Could you check a few things on this model? Use its own coordinates, in mm. Face numbers are marked on the shaded views. A direction names the side the tool comes from. Give positions to 0.01 mm unless a question says otherwise; leave off trailing zeros. Order: outer loops, then holes, each group sorted by start corner. A loop starts at its lowest first (then second) coordinate and runs counter-clockwise, first axis right, second up. Notation, with made-up numbers: M 1,-30 L 28,-30 A33 ccw 28,7 Z; hole C 89,15 d10. An arc over 180 degrees is marked long. Use a Markdown table: item, result. Add a question column.
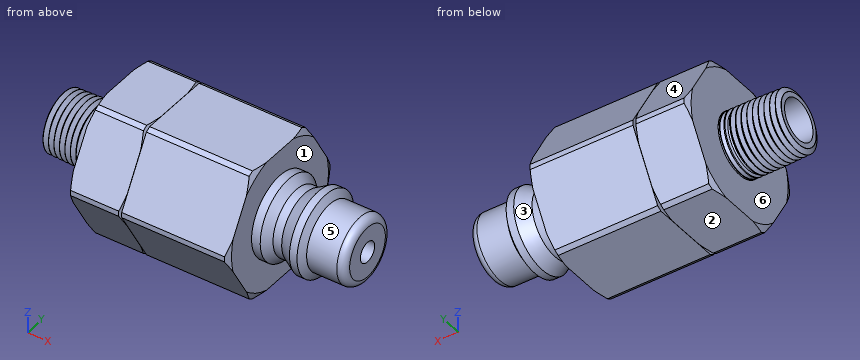
```python
from build123d import *

# Parameters (mm, degrees)
SKETCH6_W      = 11.300333551
SKETCH6_H      = 15.496408613
EXTRUDE1_DEPTH = 26.86304
FILLET1_R      = 1.27


with BuildPart() as part:
    # Sketch1 → Revolve1 (revolve)
    with BuildSketch(Plane.XY):
        Polygon((0, 0), (0, 4.202548436), (0.016953331, 4.234153018), (0.42773912, 4.999944315), (0.463586157, 5.001064591), (0.921387979, 4.262418014), (0.957235016, 4.26353829), (1.368020805, 5.029329586), (1.403867842, 5.030449862), (1.861669664, 4.291803285), (1.897516701, 4.292923561), (2.30830249, 5.058714857), (2.344149527, 5.059835133), (2.801951349, 4.321188556), (2.837798386, 4.322308832), (3.248584175, 5.088100128), (3.284431212, 5.089220404), (3.742233034, 4.350573827), (3.778080071, 4.351694103), (4.18886586, 5.1174854), (4.224712897, 5.118605675), (4.682514719, 4.379959098), (4.718361756, 4.381079374), (5.129147545, 5.146870671), (5.164994582, 5.147990947), (5.622796404, 4.409344369), (5.658643441, 4.410464645), (6.06942923, 5.176255942), (6.105276267, 5.177376218), (6.563078089, 4.43872964), (6.598925126, 4.439849916), (7.009710915, 5.205641213), (7.045557952, 5.206761489), (7.503359774, 4.468114911), (7.539206811, 4.469235187), (7.9499926, 5.235026484), (7.985839637, 5.23614676), (8.443641459, 4.497500182), (8.479488496, 4.498620458), (8.890274285, 5.264411755), (8.926121322, 5.265532031), (9.383923144, 4.526885454), (9.419770181, 4.528005729), (9.83055597, 5.293797026), (9.866403007, 5.294917302), (10.324204829, 4.556270725), (10.360051866, 4.557391001), (10.770837655, 5.323182297), (10.806684692, 5.324302573), (11.264486514, 4.585655996), (11.300333551, 4.586776272), (11.300333551, 0), align=None)
    revolve(axis=Axis((0, 0, 0), (-1, 0, 0)))

    # Sketch5 → Cut-Revolve2 (revolve, cut)
    with BuildSketch(Plane.XY, mode=Mode.PRIVATE) as cut_revolve2_sk:
        Polygon((9.96696, 0), (9.96696, 5.298059865), (11.300333551, 5.339729871), (11.300333551, 0), align=None)
    revolve(cut_revolve2_sk.sketch.rotate(Axis((0, 0, 0), (-1, 0, 0)), 180), axis=Axis((0, 0, 0), (-1, 0, 0)), mode=Mode.SUBTRACT)

    # Sketch6 → Cut-Revolve3 (revolve, cut)
    with BuildSketch(Plane.XY, mode=Mode.PRIVATE) as cut_revolve3_sk:
        with Locations((5.650166776, 12.891704307)):
            Rectangle(SKETCH6_W, SKETCH6_H)
    revolve(cut_revolve3_sk.sketch.rotate(Axis((0, 0, 0), (1, 0, 0)), 180), axis=Axis((0, 0, 0), (1, 0, 0)), mode=Mode.SUBTRACT)

    # Sketch7 → Revolve2 (revolve)
    with BuildSketch(Plane.XY, mode=Mode.PRIVATE) as revolve2_sk:
        Polygon((6.7056, 4.202548436), (9.96696, 5.1435), (9.96696, 4.202548436), align=None)
    revolve(revolve2_sk.sketch.rotate(Axis((0, 0, 0), (1, 0, 0)), 180), axis=Axis((0, 0, 0), (1, 0, 0)))

    # Sketch8 → Extrude1 (add)
    with BuildSketch(Plane(origin=(9.96696, 0, 0), x_dir=(0, 0, -1), z_dir=(1, 0, 0))):
        Polygon((0, 12.904933217), (-11.176, 6.452466608), (-11.176, -6.452466608), (0, -12.904933217), (11.176, -6.452466608), (11.176, 6.452466608), align=None)
    extrude(amount=EXTRUDE1_DEPTH)

    # Sketch9 → Cut-Revolve4 (revolve, cut)
    with BuildSketch(Plane.XY, mode=Mode.PRIVATE) as cut_revolve4_sk:
        Polygon((36.83, 11.634933217), (36.356231419, 12.650933217), (10.440728581, 12.650933217), (9.96696, 11.634933217), (9.96696, 12.904933217), (36.83, 12.904933217), align=None)
    revolve(cut_revolve4_sk.sketch.rotate(Axis((0, 0, 0), (1, 0, 0)), 180), axis=Axis((0, 0, 0), (1, 0, 0)), mode=Mode.SUBTRACT)

    # Sketch10 → Revolve3 (revolve)
    with BuildSketch(Plane.XY, mode=Mode.PRIVATE) as revolve3_sk:
        Polygon((36.83, 0), (51.562, 0), (51.562, 5.55625), (45.212, 5.55625), (44.478765158, 6.82625), (43.208765158, 6.82625), (41.009060633, 5.55625), (39.554530316, 5.55625), (38.284530316, 6.82625), (36.83, 6.82625), align=None)
    revolve(revolve3_sk.sketch.rotate(Axis((0, 0, 0), (-1, 0, 0)), 90), axis=Axis((0, 0, 0), (-1, 0, 0)))

    # Fillet1
    fillet1_edges = [part.edges().sort_by_distance(p)[0] for p in [
        (51.562, 0, 5.55625),
    ]]
    fillet(fillet1_edges, radius=FILLET1_R)

    # Sketch11 → Cut-Revolve5 (revolve, cut)
    with BuildSketch(Plane.XY):
        Polygon((11.300333551, 3.4163), (36.83, 1.70815), (51.562, 1.70815), (51.562, 0), (6.7056, 0), (0, 0), (0, 3.4163), align=None)
    revolve(axis=Axis((0, 0, 0), (-1, 0, 0)), mode=Mode.SUBTRACT)

    # Sketch12 → Cut-Revolve6 (revolve, cut)
    with BuildSketch(Plane.XY, mode=Mode.PRIVATE) as cut_revolve6_sk:
        Polygon((19.0246, 11.634933217), (18.432389274, 12.904933217), (19.05, 12.904933217), (19.05, 5.1435), (19.0246, 5.1435), align=None)
    revolve(cut_revolve6_sk.sketch.rotate(Axis((0, 0, 0), (1, 0, 0)), 270), axis=Axis((0, 0, 0), (1, 0, 0)), mode=Mode.SUBTRACT)


solid = part.part
```
1) Suppose I cut it at A-A on y = 9. Please give me the cut outline in (x, z).
2) Please list where these lines run through material, in increasing order: line 1 (Y direction, x = 7.5, z = 0); line 2 (Y direction, x = 46.5, z = 0); line 3 (Z direction, x = 3, y = -1.75). Write a range as from..to.
3) For the marked faces 4, 5 and 6, which set-ups out of +Z, -Z, +X, -X, +Y, -Y let a thin tool reach every point of the face, with its end or its side?
4) Suppose I cut it at B-B on x = 31.5. Please give me the cut outline in (y, z), and give its area (3 significant figures).
5) We'd pull the mould along X, two halves only. Please class the marked faces 1, 2 and 3: pulls with the +X half, pulls with the -X half, needs draft (parallel to the pull), parting line crosses it, or undercut.
6) Suppose I cut it at C-C on x = 12.5. Please give me the cut outline in (y, z), and give its area (3 significant figures).
7) For pin 1 (4 mm diameter, centred on x = 12.5, z = 6, fed in from -Y); pin 2 (5 mm diameter, centred on x = 41.5, y = -2.5, fed in from +Z); pin 3 (3 mm diameter, centred on y = -8, z = -2.5, fed in from -X), each with a flat end and sliding along its axis, tell me the tip position at first contact or that it passes through.
Values found:
| question | item | result |
|---|---|---|
| 1 | outline | M 9.97,-6.76 L 19.02,-6.76 L 19.02,6.76 L 9.97,6.76 Z; M 19.05,-6.76 L 36.83,-6.76 L 36.83,6.76 L 19.05,6.76 Z |
| 2 | line 1 | y = -4.47..-3.42, 3.42..4.47 |
| 2 | line 2 | y = -5.56..-1.71, 1.71..5.56 |
| 2 | line 3 | z = -4.28..-2.93, 2.93..4.28 |
| 3 | face 4 | +Z, +X, -X, +Y |
| 3 | face 5 | +X |
| 3 | face 6 | -X |
| 4 | outline | M -12.64,-0.45 L -6.71,-10.72 A12.65 ccw -5.93,-11.18 L 5.93,-11.18 A12.65 ccw 6.71,-10.72 L 12.64,-0.45 A12.65 ccw 12.64,0.45 L 6.71,10.72 A12.65 ccw 5.93,11.18 L -5.93,11.18 A12.65 ccw -6.71,10.72 L -12.64,0.45 A12.65 ccw Z; hole C 0,0 d4.13 |
| 4 | area | 419 mm^2 |
| 5 | face 1 | pulls with the +X half |
| 5 | face 2 | needs draft |
| 5 | face 3 | undercut |
| 6 | outline | M -12.64,-0.45 L -6.71,-10.72 A12.65 ccw -5.93,-11.18 L 5.93,-11.18 A12.65 ccw 6.71,-10.72 L 12.64,-0.45 A12.65 ccw 12.64,0.45 L 6.71,10.72 A12.65 ccw 5.93,11.18 L -5.93,11.18 A12.65 ccw -6.71,10.72 L -12.64,0.45 A12.65 ccw Z; hole C 0,0 d6.67 |
| 6 | area | 397 mm^2 |
| 7 | pin 1 | stops at y = -10.6 |
| 7 | pin 2 | stops at z = 6.79 |
| 7 | pin 3 | stops at x = 9.97 |
